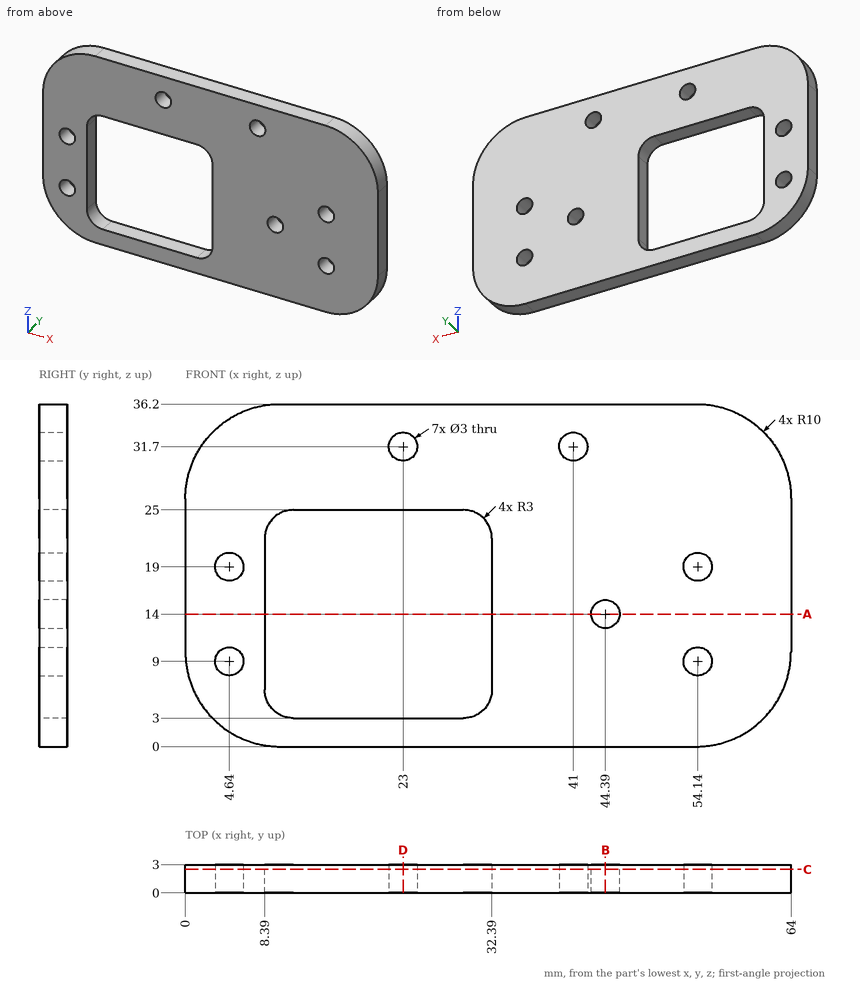
Part print with two shaded views. Sizes in mm from the minimum x, y, z corner. Round coordinates to 2 decimals unless told otherwise and drop trailing zeros. Loops run counter-clockwise (first coordinate to the right, second up) from the corner with the lowest first, then second, coordinate; pieces in that order, holes last.
1. Drill centre lines: line 1 along Z through (x, y) = (23, 1.75); line 2 along X through (y, z) = (0.85, 21.5); line 3 along X through (y, z) = (2.45, 18.5). Where is each one in solid material? Low to high.
Solutions:
line 1: z = 0 to 3, 25 to 30.2, 33.2 to 36.2
line 2: x = 0 to 8.39, 32.39 to 64
line 3: x = 0 to 3.23, 6.05 to 8.39, 32.39 to 52.73, 55.55 to 64
2. Slice it at B-B (x = 44.39). Give the cut face in (y, z).
Solutions:
outline: (0, 0) - (3, 0) - (3, 12.5) - (0, 12.5) - close; (0, 15.5) - (3, 15.5) - (3, 36.2) - (0, 36.2) - close
3. Slice it at D-D (x = 23). Give the cut face in (y, z).
Solutions:
outline: (0, 0) - (3, 0) - (3, 3) - (0, 3) - close; (0, 25) - (3, 25) - (3, 30.2) - (0, 30.2) - close; (0, 33.2) - (3, 33.2) - (3, 36.2) - (0, 36.2) - close
4. Slice it at C-C (y = 2.5). Count the separate pieces of the cut face and the enclosed holes in it, and give its area (3 significant figures).
Solutions:
separate pieces: 1
enclosed holes: 8
area: 1,660 mm2
5. Flat gauge pins, fed straight in: pin 1 (1.8 mm diameter, centred on x = 54.14, z = 19, fed in from -Y); pin 2 (5 mm diameter, centred on x = 54.14, z = 9, fed in from -Y). Where does each tip first touch, or does it go through?
Solutions:
pin 1: passes through
pin 2: stops at y = 0
6. Slice it at A-A (z = 14). Give the cut face in (x, y).
Solutions:
outline: (0, 0) - (8.39, 0) - (8.39, 3) - (0, 3) - close; (32.39, 0) - (42.89, 0) - (42.89, 3) - (32.39, 3) - close; (45.89, 0) - (64, 0) - (64, 3) - (45.89, 3) - close
